Can you work these out from the model? Positions are in its coordinate system, mm. A direction names the side the tool comes from. Give positions to 0.01 mm unless a question says otherwise; leave off trailing zeros. Loops run counter-clockwise (first coordinate to the right, second up) from the corner with the lowest first, then second, coordinate; pieces in that order, holes last. Notation, with made-up numbers: (-12, 72) -> (16, 72) arc R33 ccw to (16, 108) -> close; hole circle Ø8 at (83, 72). An arc over 180 degrees is marked (long way). Return JSON: item names as keys, results as strings. Group by question number.
Q1. Will these pins go through, and if not, where does the flat tip stop? pin 1 (0.6 mm diameter, centred on y = -14.5, z = 1, fed in from -X); pin 2 (1 mm diameter, centred on y = -49.5, z = 0.5, fed in from +X); pin 3 (12 mm diameter, centred on x = 18, y = -22, fed in from +Z); pin 4 (1 mm diameter, centred on y = 50.5, z = 0.5, fed in from -X).
Q2. Suppose I cut it at D-D, the plane y = -20. Please give me the cut outline in (x, z).
Q3. Suppose I cut it at B-B, the plane y = -39. Please give me the cut outline in (x, z), and give its area (3 significant figures).
Q4. I need wall thicknesses on line 1 along X through (y, z) = (40, 1.6); line 2 along X through (y, z) = (-28.5, 0.2); line 3 along Y through (x, z) = (45, 1.6). Which ranges of each line are inside material? Lowest first, please. Write a range as [from, to].
Q5. Which directions (+Z, -Z, +X, -X, +Y, -Y) give clear straight access to the entire face, cutting with the end or side of a thin tool? Please do faces 1 (the flat face through (-41.7, 23.7, 1)), 2 (the flat face through (-44.81, 26.31, 0.99)).
Q6. Thinking about a two-plate mould opening in Y: for faces 3 (the flat face through (41.37, 24.27, 0.99)), 4 (the flat face through (45.19, 25.65, 0.99)), 5 (the flat face through (-11.586, -20.447, 0.986)), 6 (the flat face through (-45.19, -25.65, 0.99)), which applies, pulls with the +Y half, pulls with the -Y half, needs draft (parallel to the pull), parting line crosses it, or undercut?
Q7. Suppose I cut it at A-A, the plane x = -2. Please give me the cut outline in (y, z).
Q8. Suppose I cut it at C-C, the plane x = -25.5. Please give me the cut outline in (y, z).
```python
from build123d import *

# Parameters (mm, degrees)
F1_DEPTH = 2


with BuildPart() as f1:
    # F0 (on Top) → F1 (new body)
    with BuildSketch(Plane.XY):
        Polygon((-23.5, 13.567731326), (-27.5, 11.2583302492), (-27.5, -11.2583302492), (-23.5, -13.567731326), align=None)
        Polygon((-23.5, -13.567731326), (-27.5, -11.2583302492), (-27.5, -15.8771324027), (-23.5, -18.1865334795), align=None)
        Polygon((0, -27.1354626519), (-23.5, -13.567731326), (-23.5, -18.1865334795), (-4, -29.4448637287), align=None)
        Polygon((-23.5, -18.1865334795), (-27.5, -15.8771324027), (-27.5, -43.0125950546), (-23.5, -40.7031939779), align=None)
        Polygon((-23.5, -40.7031939779), (-27.5, -43.0125950546), (-27.5, -47.6313972081), (-23.5, -45.3219961314), align=None)
        Polygon((-51, -2.3094010768), (-55, 0), (-58.75, -2.1650635095), (-31.25, -49.7964607176), (-27.5, -47.6313972081), (-27.5, -43.0125950546), (-29.7858983849, -44.3323591025), (-53.2858983849, -3.6291651246), align=None)
        Polygon((-23.5, -45.3219961314), (-27.5, -47.6313972081), (-27.5, -51.9615242271), (27.5, -51.9615242271), (27.5, -47.6313972081), (23.5, -45.3219961314), (23.5, -47.9615242271), (-23.5, -47.9615242271), align=None)
        Polygon((23.5, -40.7031939779), (4, -29.4448637287), (0, -31.7542648054), (23.5, -45.3219961314), align=None)
        Polygon((27.5, -47.6313972081), (27.5, -43.0125950546), (23.5, -40.7031939779), (23.5, -45.3219961314), align=None)
        Polygon((4, -29.4448637287), (0, -27.1354626519), (-4, -29.4448637287), (0, -31.7542648054), align=None)
        Polygon((23.5, -18.1865334795), (23.5, -13.567731326), (0, -27.1354626519), (4, -29.4448637287), align=None)
        Polygon((27.5, -15.8771324027), (27.5, -11.2583302492), (23.5, -13.567731326), (23.5, -18.1865334795), align=None)
        Polygon((58.75, -2.1650635095), (55, 0), (51, -2.3094010768), (53.2858983849, -3.6291651246), (29.7858983849, -44.3323591025), (27.5, -43.0125950546), (27.5, -47.6313972081), (31.25, -49.7964607176), align=None)
        Polygon((47, 0), (27.5, -11.2583302492), (27.5, -15.8771324027), (51, -2.3094010768), align=None)
        Polygon((-47, 0), (-51, 2.3094010768), (-55, 0), (-51, -2.3094010768), align=None)
        Polygon((-27.5, 11.2583302492), (-27.5, 15.8771324027), (-51, 2.3094010768), (-47, 0), align=None)
        Polygon((-27.5, 43.0125950546), (-27.5, 47.6313972081), (-31.25, 49.7964607176), (-58.75, 2.1650635095), (-55, 0), (-51, 2.3094010768), (-53.2858983849, 3.6291651246), (-29.7858983849, 44.3323591025), align=None)
        Polygon((-4, 29.4448637287), (-23.5, 18.1865334795), (-23.5, 13.567731326), (0, 27.1354626519), align=None)
        Polygon((-23.5, 18.1865334795), (-27.5, 15.8771324027), (-27.5, 11.2583302492), (-23.5, 13.567731326), align=None)
        Polygon((0, 31.7542648054), (-23.5, 45.3219961314), (-23.5, 40.7031939779), (-4, 29.4448637287), align=None)
        Polygon((-23.5, 45.3219961314), (-27.5, 47.6313972081), (-27.5, 43.0125950546), (-23.5, 40.7031939779), align=None)
        Polygon((27.5, 51.9615242271), (-27.5, 51.9615242271), (-27.5, 47.6313972081), (-23.5, 45.3219961314), (-23.5, 47.9615242271), (23.5, 47.9615242271), (23.5, 45.3219961314), (27.5, 47.6313972081), align=None)
        Polygon((4, 29.4448637287), (0, 31.7542648054), (-4, 29.4448637287), (0, 27.1354626519), align=None)
        Polygon((23.5, 18.1865334795), (4, 29.4448637287), (0, 27.1354626519), (23.5, 13.567731326), align=None)
        Polygon((27.5, 15.8771324027), (27.5, 43.0125950546), (23.5, 40.7031939779), (23.5, 18.1865334795), align=None)
        Polygon((27.5, 43.0125950546), (27.5, 47.6313972081), (23.5, 45.3219961314), (23.5, 40.7031939779), align=None)
        Polygon((31.25, 49.7964607176), (27.5, 47.6313972081), (27.5, 43.0125950546), (29.7858983849, 44.3323591025), (53.2858983849, 3.6291651246), (51, 2.3094010768), (55, 0), (58.75, 2.1650635095), align=None)
        Polygon((27.5, 11.2583302492), (27.5, 15.8771324027), (23.5, 18.1865334795), (23.5, 13.567731326), align=None)
        Polygon((27.5, -11.2583302492), (27.5, 11.2583302492), (23.5, 13.567731326), (23.5, -13.567731326), align=None)
        Polygon((55, 0), (51, 2.3094010768), (47, 0), (51, -2.3094010768), align=None)
    extrude(amount=F1_DEPTH)


solid = f1.part
```
Ans:
{
 "1": {"pin 1": "stops at x = -51.8", "pin 2": "stops at x = 31.71", "pin 3": "stops at z = 2", "pin 4": "stops at x = -27.5"},
 "2": {"outline": "(-48.45, 0) -> (-43.83, 0) -> (-43.83, 2) -> (-48.45, 2) -> close; (-27.5, 0) -> (-23.5, 0) -> (-23.5, 2) -> (-27.5, 2) -> close; (-20.36, 0) -> (-12.36, 0) -> (-12.36, 2) -> (-20.36, 2) -> close; (12.36, 0) -> (20.36, 0) -> (20.36, 2) -> (12.36, 2) -> close; (43.83, 0) -> (48.45, 0) -> (48.45, 2) -> (43.83, 2) -> close"},
 "3": {"outline": "(-37.48, 0) -> (-32.86, 0) -> (-32.86, 2) -> (-37.48, 2) -> close; (-27.5, 0) -> (-23.5, 0) -> (-23.5, 2) -> (-27.5, 2) -> close; (12.55, 0) -> (20.55, 0) -> (20.55, 2) -> (12.55, 2) -> close; (32.86, 0) -> (37.48, 0) -> (37.48, 2) -> (32.86, 2) -> close", "area": "42.5 mm^2"},
 "4": {"line 1": "x = [-36.91, -32.29], [-22.28, -14.28], [23.5, 27.5], [32.29, 36.91]", "line 2": "x = [-43.55, -38.93], [-27.5, -23.5], [-5.64, 5.64], [38.93, 43.55]", "line 3": "y = [-25.98, -17.98], [-5.77, -1.15], [17.98, 25.98]"},
 "5": {"face 1": "+Z, -Z", "face 2": "+Z, -Z, -X, +Y"},
 "6": {"face 3": "undercut", "face 4": "pulls with the +Y half", "face 5": "undercut", "face 6": "pulls with the -Y half"},
 "7": {"outline": "(-51.96, 0) -> (-47.96, 0) -> (-47.96, 2) -> (-51.96, 2) -> close; (-30.6, 0) -> (-25.98, 0) -> (-25.98, 2) -> (-30.6, 2) -> close; (25.98, 0) -> (32.91, 0) -> (32.91, 2) -> (25.98, 2) -> close; (47.96, 0) -> (51.96, 0) -> (51.96, 2) -> (47.96, 2) -> close"},
 "8": {"outline": "(-51.96, 0) -> (17.03, 0) -> (17.03, 2) -> (-51.96, 2) -> close; (41.86, 0) -> (51.96, 0) -> (51.96, 2) -> (41.86, 2) -> close"}
}
